Here's the drawing with two shaded views (mm, measured from the low corner). I have some questions. Coordinates: 2 decimals unless noted, no trailing zeros. Write each loop counter-clockwise with the first axis right and the second up, starting at its lowest first coordinate (ties: lowest second). Pieces come first, ordered by that corner, then holes. Notation, with made-up numbers: (45.5, 8) -> (65.5, 8) arc R22 cw to (65.5, 16) -> close; hole circle Ø7 at (36.25, 80). An arc over 180 degrees is marked (long way). Put each result on its own line as item: value.
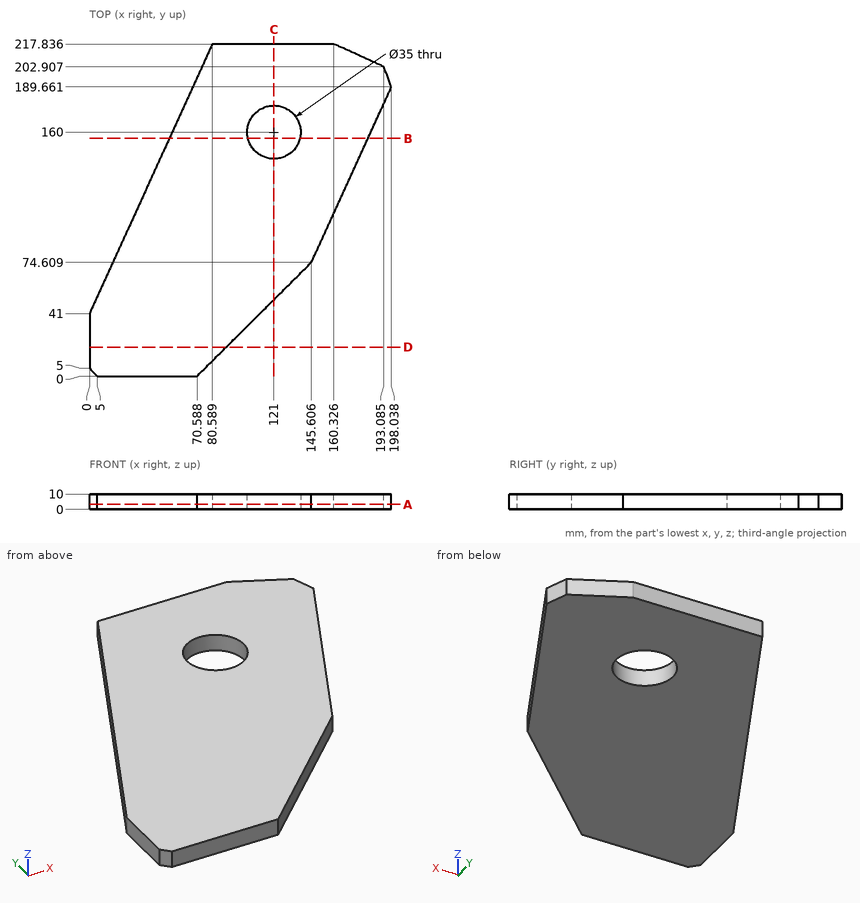
Item 1: Imagine slicing it at D-D on y = 19. Write out the boundary of the cut face in (x, z).
Output:
outline: (0, 0) -> (89.69, 0) -> (89.69, 10) -> (0, 10) -> close
Item 2: Imagine slicing it at B-B on y = 156. Write out the boundary of the cut face in (x, z), then the cut area to 3 significant figures.
Output:
outline: (52.41, 0) -> (103.96, 0) -> (103.96, 10) -> (52.41, 10) -> close; (138.04, 0) -> (182.7, 0) -> (182.7, 10) -> (138.04, 10) -> close
area: 962 mm²
Item 3: Please list where these lines run through material, in increasing order: line 1 along Y through (x, z) = (107, 3) (1 decimal); line 2 along X through (y, z) = (168, 9.25) (1 decimal); line 3 along Y through (x, z) = (121, 3) (1 decimal). Write a range as from..to.
Output:
line 1: y = 36.2..149.5, 170.5..217.8
line 2: x = 57.9..105.4, 136.6..188.2
line 3: y = 50.1..142.5, 177.5..217.8
Item 4: For P1, Ø3, axis at x = 78, z = 2, coming from the -Y side; P2, Ø1, axis at x = 127, z = 2, coming from the -Y side; P3, Ø3, axis at x = 148.5, z = 4, coming from the -Y side, each with a flat end and sliding along its axis, tell me the tip position at first contact or that it passes through.
Output:
P1: stops at y = 5.88
P2: stops at y = 55.61
P3: stops at y = 77.67
Item 5: Imagine slicing it at A-A on z = 3.25. Write out the boundary of the cut face in (x, y) (1 decimal), then the cut area to 3 significant figures.
Output:
outline: (0, 5) -> (5, 0) -> (70.6, 0) -> (145.6, 74.6) -> (198, 189.7) -> (193.1, 202.9) -> (160.3, 217.8) -> (80.6, 217.8) -> (0, 41) -> close; hole circle Ø35 at (121, 160)
area: 25,000 mm²
Item 6: Imagine slicing it at C-C on x = 121. Write out the boundary of the cut face in (y, z).
Output:
outline: (50.14, 0) -> (142.5, 0) -> (142.5, 10) -> (50.14, 10) -> close; (177.5, 0) -> (217.84, 0) -> (217.84, 10) -> (177.5, 10) -> close
